Source: CAD feature listing. Evaluate the final solid. Frame: model axes, mm. A direction names the side the tool comes from. Round coordinates to 2 decimals unless told otherwise and drop trailing zeros. Order: outer loops, then holes, each group sorted by start corner. A loop starts at its lowest first (then second) coordinate and runs counter-clockwise, first axis right, second up. Notation, with made-up numbers: (-0.5, 16) -> (15.5, 16) arc R19 ccw to (15.5, 24) -> close; hole circle Ø8 at (-8.75, -30.75). An arc over 180 degrees is marked (long way). Answer as CSV lines item,"result".
from build123d import *

# Parameters (mm, degrees)
SKETCH1_R                = 22.225
HUB_CENTER_DEPTH         = 25.4
HUB_CENTER_DEPTH_BACK    = 23.4
INNER_START              = 1.397
SKETCH2_R                = 29.21
INNER_BEARING_DEPTH      = 13.208
OUTER_START              = -1.397
SKETCH3_R                = 29.21
OUTER_BEARING_DEPTH      = 13.208
TIRE_ARM_DEPTH           = 2.54
SKETCH5_W                = 25.4
SKETCH5_H                = 152.4
TIRE_CONTACT_PATCH_DEPTH = 2.54


with BuildPart() as part:
    # Sketch1 → Hub Center (new body, two sides)
    with BuildSketch(Plane.XY) as hub_center_sk:
        Circle(SKETCH1_R)
    extrude(amount=HUB_CENTER_DEPTH)
    extrude(hub_center_sk.sketch, amount=-HUB_CENTER_DEPTH_BACK)

    # Sketch2 → Inner Bearing (add)
    with BuildSketch(Plane.XY.offset(INNER_START)):
        Circle(SKETCH2_R)
    extrude(amount=INNER_BEARING_DEPTH)

    # Sketch3 → Outer Bearing (add)
    with BuildSketch(Plane.XY.offset(OUTER_START)):
        Circle(SKETCH3_R)
    extrude(amount=-OUTER_BEARING_DEPTH)

    # Sketch4 → Tire Arm (add)
    with BuildSketch(Plane(origin=(0, 0, -23.4), x_dir=(-1, 0, 0), z_dir=(0, 0, -1))):
        with BuildLine():
            Line((-12.7, -18.238986403), (-12.7, -266.7))
            Line((-12.7, -266.7), (12.7, -266.7))
            Line((12.7, -266.7), (12.7, -18.238986403))
            ThreePointArc((12.7, -18.238986403), (0, -22.225), (-12.7, -18.238986403))
        make_face()
    extrude(amount=-TIRE_ARM_DEPTH)

    # Sketch5 → Tire Contact Patch (add)
    with BuildSketch(Plane.XZ.offset(266.7)):
        with Locations((0, -22.13)):
            Rectangle(SKETCH5_W, SKETCH5_H)
    extrude(amount=-TIRE_CONTACT_PATCH_DEPTH)


solid = part.part
1. Section query D-D on x = 25. Return loops of the section in (y, z) (3 decimals).
Results below:
outline,"(-15.107, -14.605) -> (15.107, -14.605) -> (15.107, -1.397) -> (-15.107, -1.397) -> close; (-15.107, 1.397) -> (15.107, 1.397) -> (15.107, 14.605) -> (-15.107, 14.605) -> close"
2. Section query B-B on y = 0. Return loops of the section in (x, z) (3 decimals).
Results below:
outline,"(-29.21, -14.605) -> (-22.225, -14.605) -> (-22.225, -23.4) -> (22.225, -23.4) -> (22.225, -14.605) -> (29.21, -14.605) -> (29.21, -1.397) -> (22.225, -1.397) -> (22.225, 1.397) -> (29.21, 1.397) -> (29.21, 14.605) -> (22.225, 14.605) -> (22.225, 25.4) -> (-22.225, 25.4) -> (-22.225, 14.605) -> (-29.21, 14.605) -> (-29.21, 1.397) -> (-22.225, 1.397) -> (-22.225, -1.397) -> (-29.21, -1.397) -> close"
3. Line query: L1, parallel to Y at x = -1, z = 8; L2, parallel to Z at x = 18, y = -17.5 (3 decimals); L3, parallel to Y at x = -6, z = 44.5. Output: solid intervals per line, ascending. Write a range as [from, to].
Results below:
L1,"[-266.7, -264.16], [-29.19, 29.19]"
L2,"[-14.605, -1.397], [1.397, 14.605]"
L3,"[-266.7, -264.16]"
4. Mould query, pull axis Y, two halves, no side actions, for faces 1 (the cylindrical face through (21.199, 6.676, 20.078)), 2 (the flat face through (0, -266.7, -21)), 3 (the flat face through (0, -139, -20.86)), 4 (the flat face through (0, 0, 25.4)). Classes: released by +Y, released by -Y, zero draft, split by the parting line, or undercut.
Results below:
face 1,"undercut"
face 2,"released by -Y"
face 3,"undercut"
face 4,"zero draft"
5. Pin query (flat end, axial travel): pin 1 (8 mm diameter, centred on x = -16, z = 28.5, fed in from +Y); pin 2 (22 mm diameter, centred on x = -6.5, y = -139.5, fed in from -Z); pin 3 (6 mm diameter, centred on x = -5.5, y = -54, fed in from +Z); pin 4 (1 mm diameter, centred on x = 21.5, z = 26.5, fed in from -Y). Return the tip coordinate at first contact, or that it passes through.
Results below:
pin 1,"y = 17.68"
pin 2,"z = -23.4"
pin 3,"z = -20.86"
pin 4,"through"
6. Reachability of faces 5 (the cylindrical face through (21.199, 6.676, 0.02)), 6 (the flat face through (0, -264.16, 17)), 7 (the flat face through (-11, 20, 14.605)), 8 (the flat face through (0, -264.16, -60)) from +Z, -Z, +X, -X, +Y, -Y: full face, straight path, thin tool, end or side. Return the list, or none.
Results below:
face 5,"none"
face 6,"+Z, +X, -X"
face 7,"+Z"
face 8,"-Z, +X, -X, +Y"
7. Section query A-A on z = -6.5. Return loops of the section in (x, y), and give its area (4 significant figures).
Results below:
outline,"circle Ø58.42 at (0, 0); (-12.7, -266.7) -> (12.7, -266.7) -> (12.7, -264.16) -> (-12.7, -264.16) -> close"
area,"2,745 mm2"
8. Section query C-C on x = 0. Return loops of the section in (y, z) (3 decimals), and give its area (3 significant figures).
Results below:
outline,"(-266.7, -98.33) -> (-264.16, -98.33) -> (-264.16, -23.4) -> (22.225, -23.4) -> (22.225, -14.605) -> (29.21, -14.605) -> (29.21, -1.397) -> (22.225, -1.397) -> (22.225, 1.397) -> (29.21, 1.397) -> (29.21, 14.605) -> (22.225, 14.605) -> (22.225, 25.4) -> (-22.225, 25.4) -> (-22.225, 14.605) -> (-29.21, 14.605) -> (-29.21, 1.397) -> (-22.225, 1.397) -> (-22.225, -1.397) -> (-29.21, -1.397) -> (-29.21, -14.605) -> (-22.225, -14.605) -> (-22.225, -20.86) -> (-264.16, -20.86) -> (-264.16, 54.07) -> (-266.7, 54.07) -> close"
area,"3,540 mm2"
